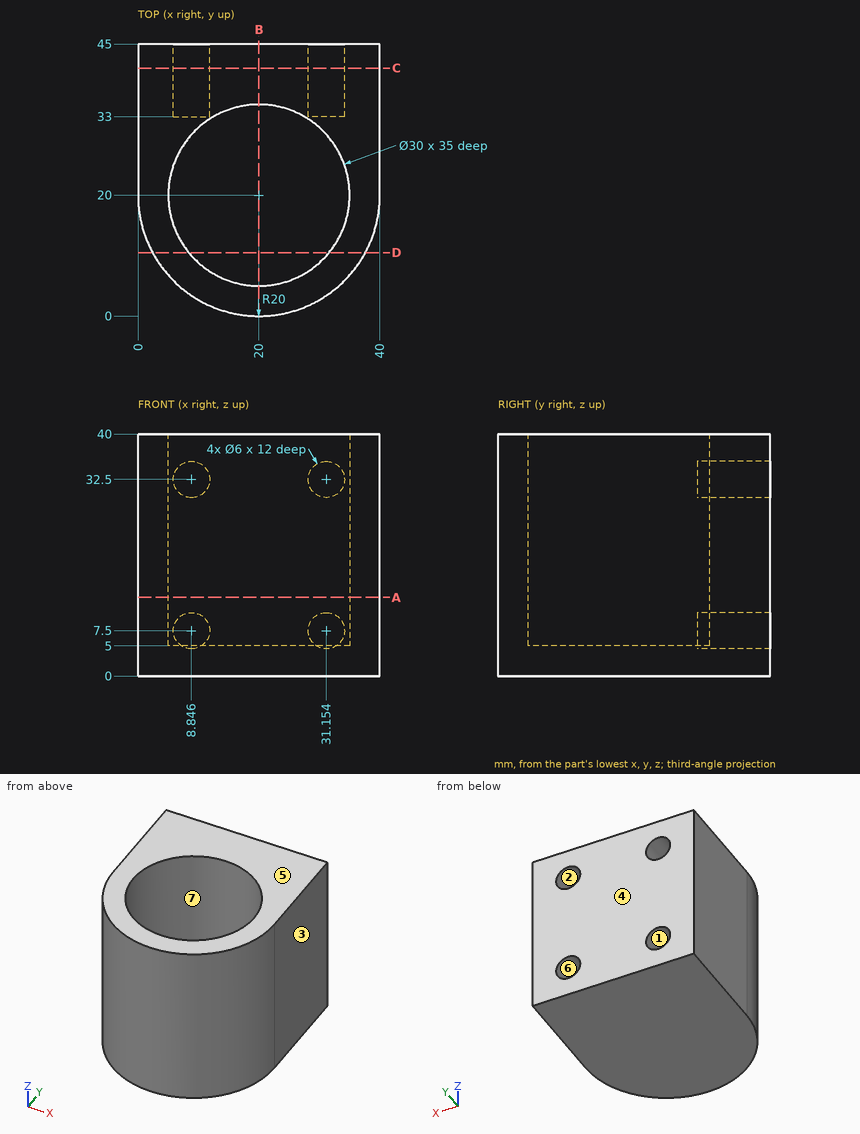
Print and shaded views of the part. All mm, measured from the part's lowest x, y and z. A direction names the side the tool comes from. Give positions to 0.01 mm unless a question says otherwise; leave off trailing zeros. Order: outer loops, then holes, each group sorted by start corner. A loop starts at its lowest first (then second) coordinate and runs counter-clockwise, first axis right, second up. Notation, with made-up numbers: (34.5, -11.75) - (79.5, -11.75) arc R18 ccw to (79.5, 15.25) - close; hole circle Ø7 at (68, -33). An arc over 180 degrees is marked (long way). One line per item, written item: value.
Item 1: Slice it at A-A (z = 13). List the corners of the cut face in (x, y), then the cut area to 3 significant figures.
Response values:
outline: (0, 20) arc R20 ccw to (40, 20) - (40, 45) - (0, 45) - close; hole circle Ø30 at (20, 20)
area: 921 mm2
Item 2: Slice it at B-B (x = 20). List the corners of the cut face in (y, z), then the cut area to 3 significant figures.
Response values:
outline: (0, 0) - (45, 0) - (45, 40) - (35, 40) - (35, 5) - (5, 5) - (5, 40) - (0, 40) - close
area: 750 mm2
Item 3: Two-plate mould, pull along X, no slides. Class the marked faces 1, 2, 3 and 4: released by +X, released by -X, zero draft, split by the parting line, or undercut.
Response values:
face 1: undercut
face 2: undercut
face 3: released by +X
face 4: zero draft
Item 4: Wall check: line 1 (X direction, y = 38, z = 7.5); line 2 (Z direction, x = 32, y = 38); line 3 (Z direction, x = 32, y = 26.5). Give the ranges that are in metal, low to high.
Response values:
line 1: 0 to 5.85, 11.85 to 28.15, 34.15 to 40
line 2: 0 to 4.62, 10.38 to 29.62, 35.38 to 40
line 3: 0 to 5
Item 5: Slice it at C-C (y = 41). List the corners of the cut face in (x, z).
Response values:
outline: (0, 0) - (40, 0) - (40, 40) - (0, 40) - close; hole circle Ø6 at (8.85, 7.5); hole circle Ø6 at (8.85, 32.5); hole circle Ø6 at (31.15, 7.5); hole circle Ø6 at (31.15, 32.5)
Item 6: Tool access for the marked faces 5, 6 and 7: list every direction of +Z, -Z, +X, -X, +Y, -Y with a clear straight run to the whole face (end or side of a thin tool).
Response values:
face 5: +Z, +X, -X, +Y, -Y
face 6: +Y
face 7: +Z
Item 7: Slice it at D-D (y = 10.5). List the corners of the cut face in (x, z).
Response values:
outline: (2.4, 0) - (37.6, 0) - (37.6, 40) - (31.61, 40) - (31.61, 5) - (8.39, 5) - (8.39, 40) - (2.4, 40) - close
Item 8: Pin check, flat tips, straight feed: pin 1 Ø3 at (x, z) = (9, 7) entering from +Y; pin 2 Ø3.5 at (x, z) = (8.85, 7.5) entering from -Y; pin 3 Ø24 at (x, y) = (20, 20) entering from +Z. Stop position of each tip, or through.
Response values:
pin 1: y = 33
pin 2: y = 2.35
pin 3: z = 5
